```python
from build123d import *

# Parameters (mm, degrees)
F0_W     = 6
F0_H     = 214
F0_H_2   = 6
F0_W_2   = 44
F1_DEPTH = 100
F3_D     = 7
F4_W     = 47
F4_H     = 50
F5_DEPTH = 25


with BuildPart() as f1:
    # F0 (on Right) → F1 (new body)
    with BuildSketch(Plane.YZ):
        with Locations((-3, 113)):
            Rectangle(F0_W, F0_H)
        with Locations((-3, 3)):
            Rectangle(F0_W, F0_H_2)
        with Locations((-28, 3)):
            Rectangle(F0_W_2, F0_H_2)
    extrude(amount=F1_DEPTH)

    # F3 (through all)
    with Locations(Plane(origin=(0, 0, 0), x_dir=(1, 0, 0), z_dir=(0, 0, -1))):
        with Locations((30, 41.0281047225), (90, 41.0281047225)):
            Hole(F3_D / 2)

    # F4 (on Front) → F5 (cut)
    with BuildSketch(Plane.XZ):
        with Locations((43.5, 195)):
            Rectangle(F4_W, F4_H)
    extrude(amount=F5_DEPTH, mode=Mode.SUBTRACT)


with BuildPart() as f6_1:
    # F6: instance of F1
    add(f1.part.mirror(Plane.XZ))


with BuildPart() as f8_1:
    # F8: instance of F1
    add(f1.part.mirror(Plane.XZ))


solid = f8_1.part
```
Can you work these out from the model? Positions are in its coordinate system, mm. A direction names the side the tool comes from. Round coordinates to 2 decimals unless told otherwise and drop trailing zeros. Loops run counter-clockwise (first coordinate to the right, second up) from the corner with the lowest first, then second, coordinate; pieces in that order, holes last. Notation, with made-up numbers: (27.25, -15.5) -> (86.25, -15.5) arc R21 cw to (86.25, 5.5) -> close; hole circle Ø3 at (59, 73.5). An arc over 180 degrees is marked (long way). Answer in a Markdown table with one row per item.
Item 1: Will these pins go through, and if not, where does the flat tip stop? P1, Ø3, axis at x = 49, y = 3, coming from the +Z side; P2, Ø5.5, axis at x = 90, y = 41.03, coming from the -Z side; P3, Ø4, axis at x = 41.5, y = 20.5, coming from the +Z side; P4, Ø6, axis at x = 80.5, z = 114, coming from the -Y side.
Answer block:
| item | result |
|---|---|
| P1 | z = 170 |
| P2 | through |
| P3 | z = 6 |
| P4 | y = 0 |
Item 2: If I drill on probe 1 along X at (y, z) = (4.5, 191); probe 2 along Y at (x, z) = (30, 4); probe 3 along Y at (x, z) = (35.5, 61.5), over which ranges is the centre line in solid material (lowest first)?
Answer block:
| item | result |
|---|---|
| probe 1 | 0 to 20, 67 to 100 |
| probe 2 | 0 to 37.53, 44.53 to 50 |
| probe 3 | 0 to 6 |
Item 3: Suppose I cut it at D-D, the plane z = 57.5. List the corners of the cut face in (x, y) for me, plus the area to 3 significant figures.
Answer block:
| item | result |
|---|---|
| outline | (0, 0) -> (100, 0) -> (100, 6) -> (0, 6) -> close |
| area | 600 mm² |
Item 4: Suppose I cut it at C-C, the plane x = 40. List the corners of the cut face in (y, z) for me.
Answer block:
| item | result |
|---|---|
| outline | (0, 0) -> (50, 0) -> (50, 6) -> (6, 6) -> (6, 170) -> (0, 170) -> close |
Item 5: Suppose I cut it at A-A, the plane x = 30. List the corners of the cut face in (y, z) for me.
Answer block:
| item | result |
|---|---|
| outline | (0, 0) -> (37.53, 0) -> (37.53, 6) -> (6, 6) -> (6, 170) -> (0, 170) -> close; (44.53, 0) -> (50, 0) -> (50, 6) -> (44.53, 6) -> close |
Item 6: On a 3-axis mill with a long thin cutter (end or side, diameter ignored), from which of +Z, -Z, +X, -X, +Y, -Y can I reach the whole of each face in a straight line? I mean faces 1 (the flat face through (49, 50, 3)), 2 (the flat face through (20, 3, 195)), 3 (the flat face through (49, 28, 6)). Say none if no direction works.
Answer block:
| item | result |
|---|---|
| face 1 | +Z, -Z, +X, -X, +Y |
| face 2 | +Z, +Y, -Y |
| face 3 | +Z, +X, -X, +Y |
Item 7: We'd pull the mould along Y, two halves only. Please class faces 4 (the flat face through (0, 3, 86)), 5 (the cylindrical face through (86.66, 42.08, 3.04)), 6 (the flat face through (49, 6, 114)): released by +Y, released by -Y, zero draft, split by the parting line, or undercut.
Answer block:
| item | result |
|---|---|
| face 4 | zero draft |
| face 5 | undercut |
| face 6 | released by +Y |
Item 8: Suppose I cut it at B-B, the plane z = 200.5. List the corners of the cut face in (x, y) for me.
Answer block:
| item | result |
|---|---|
| outline | (0, 0) -> (20, 0) -> (20, 6) -> (0, 6) -> close; (67, 0) -> (100, 0) -> (100, 6) -> (67, 6) -> close |
